from build123d import *

# Parameters (mm, degrees)
F0_W     = 38.1
F0_H     = 889
F1_DEPTH = 38.1
F3_DEPTH = 38.101


with BuildPart() as f1:
    # F0 (on Front) → F1 (new body)
    with BuildSketch(Plane.XZ):
        with Locations((19.05, 444.5)):
            Rectangle(F0_W, F0_H)
    extrude(amount=F1_DEPTH)

    # F2 (on face) → F3 (cut, through all)
    with BuildSketch(Plane(origin=(0, 0, 0), x_dir=(0, -1, 0), z_dir=(-1, 0, 0))):
        Polygon((38.1, 889), (3.175, 889), (38.1, 854.075), align=None)
        Polygon((38.1, 34.925), (3.175, 0), (38.1, 0), align=None)
    extrude(amount=-F3_DEPTH, mode=Mode.SUBTRACT)


solid = f1.part
Build history of the part. All positions in model axes, mm. Coordinates: 2 decimals unless noted, no trailing zeros. Write each loop counter-clockwise with the first axis right and the second up, starting at its lowest first coordinate (ties: lowest second). Pieces come first, ordered by that corner, then holes.
(1) Cut at A-A on x = 21. List the corners of the cut face in (y, z) (3 decimals), and give its area (3 significant figures).
(2) Cut at B-B on y = -19. List the corners of the cut face in (x, z) (3 decimals).
(3) Pin check, flat tips, straight feed: pin 1 Ø12 at (x, y) = (25.5, -33) entering from +Z (3 decimals); pin 2 Ø5 at (x, y) = (21.5, -32.5) entering from -Z (3 decimals); pin 3 Ø12 at (x, y) = (24, -22) entering from +Z (3 decimals). Stop position of each tip, or through.
(4) Drill centre lines: line 1 (Z direction, x = 4, y = -11) (3 decimals); line 2 (Z direction, x = 11, y = -7) (3 decimals). Where is each one in solid material? Low to high.
Working result:
1. outline: (-38.1, 34.925) - (-3.175, 0) - (0, 0) - (0, 889) - (-3.175, 889) - (-38.1, 854.075) - close
1. area: 32,700 mm2
2. outline: (0, 15.825) - (38.1, 15.825) - (38.1, 873.175) - (0, 873.175) - close
3. pin 1: stops at z = 865.175
3. pin 2: stops at z = 26.825
3. pin 3: stops at z = 876.175
4. line 1: z = 7.825 to 881.175
4. line 2: z = 3.825 to 885.175
